Here's the drawing with two shaded views (mm, measured from the low corner). I have some questions. Give positions to 0.01 mm unless a question says otherwise; leave off trailing zeros. Loops run counter-clockwise (first coordinate to the right, second up) from the corner with the lowest first, then second, coordinate; pieces in that order, holes last. Notation, with made-up numbers: (86.5, -6.75) - (93.5, -6.75) arc R14 ccw to (93.5, 20.25) - close; hole circle Ø8 at (66, 16.25). An arc over 180 degrees is marked (long way). Write each question's results on one line, items separated by ' | '. Start each with the question number.
1) I'm going to push flat-ended pins straight in: pin 1 (1.5 mm diameter, centred on y = 1.5, z = 22, fed in from -X); pin 2 (0.9 mm diameter, centred on y = 2, z = 79, fed in from +X); pin 3 (1 mm diameter, centred on x = 41, z = 45, fed in from -Y); pin 4 (10 mm diameter, centred on x = 64, z = 26.5, fed in from -Y). Where does each tip first touch, or does it pass through?
2) If I drill on probe 1 along Z at (x, y) = (5, 2.1); probe 2 along X at (y, z) = (2.15, 61.5); probe 3 along Z at (x, y) = (4.5, 1.9), over which ranges is the centre line in solid material (lowest first)? Write a range as [from, to].
3) I want a section at D-D, the plane x = 17.5. Write out the boundary of the cut face in (y, z), and give its area (3 significant figures).
4) I want a section at B-B, the plane z = 48.5. Write out the boundary of the cut face in (x, y).
5) I want a section at C-C, the plane y = 0.8. Count the separate pieces of the cut face and the enclosed holes in it, and give its area (3 significant figures).
6) I want a section at A-A, the plane x = 5. Write out the boundary of the cut face in (y, z), and give its area (3 significant figures).
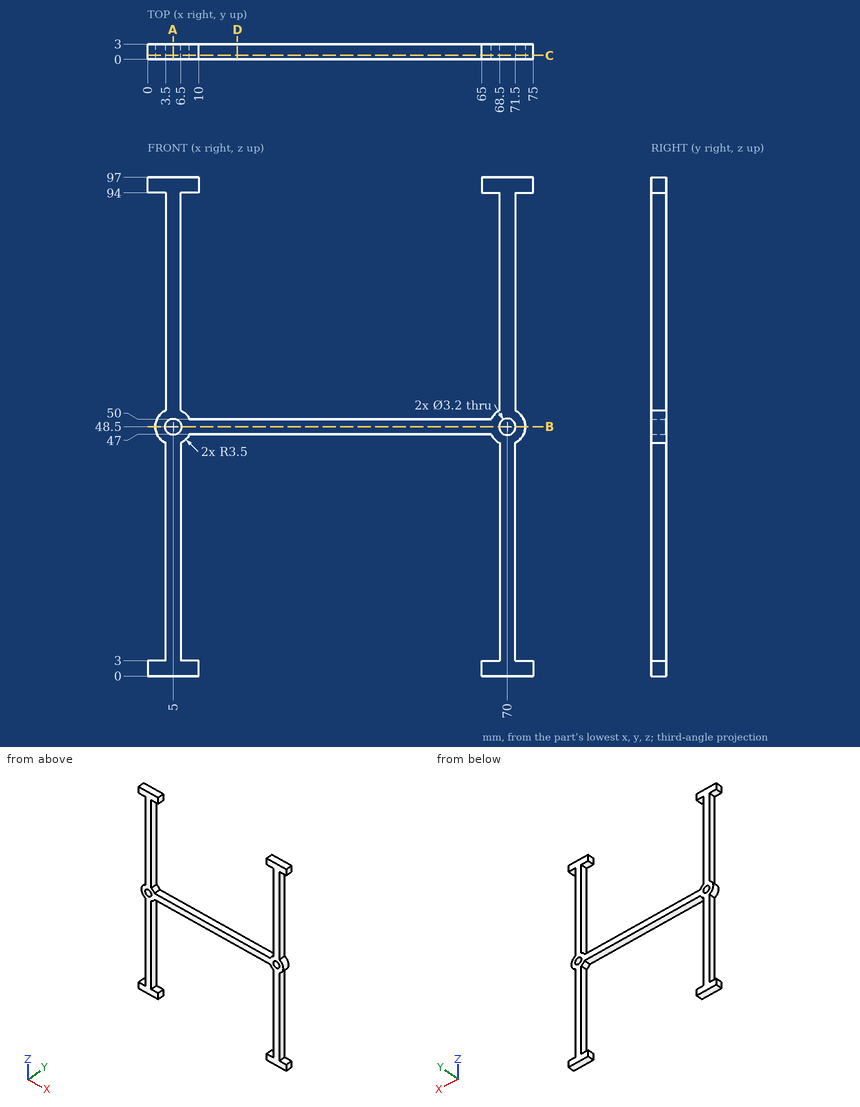
Answers:
1) pin 1: stops at x = 3.5 | pin 2: stops at x = 71.5 | pin 3: passes through | pin 4: stops at y = 0
2) probe 1: z = [0, 46.9], [50.1, 97] | probe 2: x = [3.5, 6.5], [68.5, 71.5] | probe 3: z = [0, 46.98], [50.02, 97]
3) outline: (0, 47) - (3, 47) - (3, 50) - (0, 50) - close | area: 9.00 mm2
4) outline: (1.5, 0) - (3.4, 0) - (3.4, 3) - (1.5, 3) - close; (6.6, 0) - (68.4, 0) - (68.4, 3) - (6.6, 3) - close; (71.6, 0) - (73.5, 0) - (73.5, 3) - (71.6, 3) - close
5) separate pieces: 1 | enclosed holes: 2 | area: 861 mm2
6) outline: (0, 0) - (3, 0) - (3, 46.9) - (0, 46.9) - close; (0, 50.1) - (3, 50.1) - (3, 97) - (0, 97) - close | area: 281 mm2
